Autodesk Inventor part; units mm, degrees
ref_plane "YZ Plane" through (0, 0, 0) normal (1, 0, 0) x (0, 1, 0)
ref_plane "XZ Plane" through (0, 0, 0) normal (0, 1, 0) x (-1, 0, 0)
ref_plane "XY Plane" through (0, 0, 0) normal (0, 0, 1) x (1, 0, 0)
sketch "草图1" plane through (0, 0, 0) normal (0, 0, 1) x (1, 0, 0)
  circle A0 centre (0, 0) radius 2.8
  circle A1 centre (0, 0) radius 1 construction
  line L0 (0, 2.8) -> (0, 2.4)
  line L1 (0, 2.4) -> (0.3748, 2.7748)
  line L2 (0, 2.4) -> (-0.3748, 2.7748)
  line L3 (0, 2.4) -> (0.53, 2.4) construction
  line L4 (0, 0) -> (0, 2.8) construction
  line L5 (0, 0) -> (-2.8, 0) construction
  line L6 (0, 0) -> (0, -2.8) construction
  circle A2 centre (0, 1) radius 0.225
  circle A3 centre (0, -1) radius 0.225
  circle A4 centre (-1, 0) radius 0.225
  circle A5 centre (-1, 0) radius 0.6
  line L7 (0, -2.8) -> (0, -2.4)
  line L8 (0, -2.4) -> (0.3748, -2.7748)
  line L9 (0, -2.4) -> (-0.3748, -2.7748)
  line L10 (0, -2.4) -> (0.53, -2.4) construction
  line L11 (-2.4, 0) -> (-2.4, 0.5)
  line L12 (-2.4, 0.5) -> (-2.755, 0.5)
  line L13 (-2.4, 0) -> (-2.4, -0.5)
  line L14 (-2.4, -0.5) -> (-2.755, -0.5)
  point P0 (-0.3748, -2.7748)
  point P1 (0.3748, -2.7748)
  dimension "d0" = 5.6
  dimension "d1" = 2
  dimension "d5" = 0.4
  dimension "d6" = 45
  dimension "d7" = 135
  dimension "d8" = 0.45
  dimension "d9" = 0.45
  dimension "d10" = 0.45
  dimension "d11" = 1.2
  dimension "d12" = 0.5
  dimension "d13" = 0.5
  dimension "d14" = 0.4
extrude "拉伸1" add sketch "草图1" along normal blind 1.2 contours A0 L8 L9 L14 L13 L11 L12 L2 L1 | A2 | A3 | A4 | A5
extrude "拉伸2" add sketch "草图1" against normal blind 6.5 contours A2 | A3 | A4
extrude "拉伸3" add sketch "草图1" against normal blind 0.5 contours A5
sketch "草图2" plane through (0, 0, 1.2) normal (0, 0, 1) x (1, 0, 0)
  circle A0 centre (0, 0) radius 1.8
  circle A1 centre (0, 0) radius 2.2
  dimension "d21" = 3.6
  dimension "d22" = 4.4
extrude "拉伸4" add sketch "草图2" along normal blind 2.37 contours A0
extrude "拉伸5" add sketch "草图2" along normal blind 0.3
sketch "草图3" plane through (0, 0, 0) normal (1, 0, 0) x (0, 1, 0)
  line L0 (1.8, 3.57) -> (-1.8, 3.57)
  line L1 (0, 3.57) -> (-0.8, 3.57)
  line L2 (-0.8, 3.57) -> (-0.5879, 3.3579)
  line L3 (-0.5879, 3.3579) -> (0, 3.3579)
  line L4 (0, 3.3579) -> (0, 3.57)
  point P0 (0, 0)
  dimension "d27" = 0.8
  dimension "d28" = 0.3
  dimension "d29" = 45
revolve "旋转1" cut sketch "草图3" angle 360 about axis through (0, 0, 3.3579) along (0, 0, 1)
fillet "圆角1" radius 0.25 2 edges at (-1.8, 0, 3.57) (-1.8, 0, 1.5)
properties part number "CAN_φ5.6" material "黄铜，软黄"
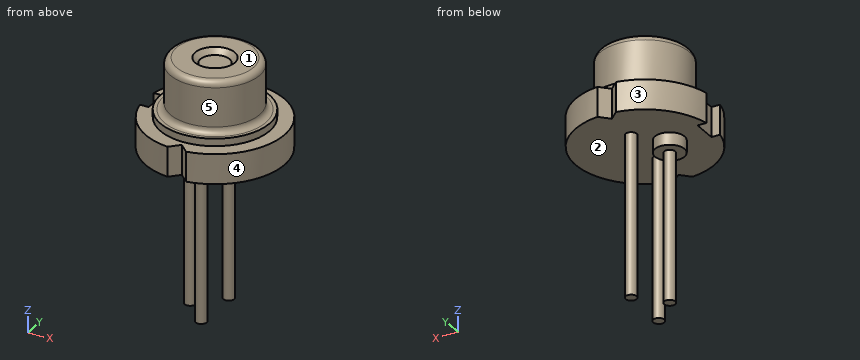
Can you work these out from the model? Positions are in its coordinate system, mm. Face numbers are marked on the shaded views. A direction names the side the tool comes from. Give positions to 0.01 mm unless a question says otherwise; leave off trailing zeros. Loops run counter-clockwise (first coordinate to the right, second up) from the corner with the lowest first, then second, coordinate; pieces in that order, holes last. Notation, with made-up numbers: M 85.5,72.5 L 94.5,72.5 A22 cw 94.5,94.5 Z; hole C -36,37.25 d4. An arc over 180 degrees is marked long. One line per question, with ' | ' between items. Start each with the question number.
Q1. If we section it at A-A (z = -2.25): Please give me the cut outline in (x, y) (3 decimals).
Q2. If we mould it in two halves opening along Z, with no side actions, what happens to the marked faces 1, 2 and 3? For each: +Z half, -Z half, draft (parallel to the pull), parting line (faces both ways), or undercut.
Q3. If I drill on line 1 (Z direction, x = -1.9, y = -0.1); line 2 (Z direction, x = 0.8, y = 2.4); line 3 (X direction, y = -0.85, z = 2.75), over which ranges is the centre line in solid material (lowest first)? Write a range as from..to.
Q4. For pin 1 Ø0.9 at (x, y) = (0, 0) entering from +Z; pin 2 Ø2 at (x, y) = (-2, 1.5) entering from -Z, each with a flat end and sliding along its axis, tell me the tip position at first contact or that it passes through.
Q5. For the marked faces 4 and 5, which set-ups out of +Z, -Z, +X, -X, +Y, -Y let a thin tool reach every point of the face, with its end or its side?
Computed:
1) outline: C -1,0 d0.45; C 0,-1 d0.45; C 0,1 d0.45
2) face 1: +Z half | face 2: -Z half | face 3: draft
3) line 1: z = 0..1.55 | line 2: z = 0..1.2 | line 3: x = -1.59..1.59
4) pin 1: stops at z = 3.36 | pin 2: stops at z = 0
5) face 4: +Z, -Z, +X | face 5: +Z
